from build123d import *

# Parameters (mm, degrees)
SKETCH1_R           = 8.75
BOSS_EXTRUDE1_DEPTH = 180
SKETCH2_R           = 8.75
SKETCH2_R_2         = 8
CUT_EXTRUDE1_DEPTH  = 40.95
CUT_EXTRUDE2_DEPTH  = 33.8
CUT_EXTRUDE3_DEPTH  = 33.8
CUT_EXTRUDE4_DEPTH  = 33.8
SKETCH7_R           = 8.75
BOSS_EXTRUDE2_DEPTH = 7.8
SKETCH9_R           = 8.75
BOSS_EXTRUDE3_DEPTH = 0.3
BOSS_EXTRUDE3_TAPER = 75


with BuildPart() as part:
    # Sketch1 → Boss-Extrude1 (new body)
    with BuildSketch(Plane.XY):
        Circle(SKETCH1_R)
    extrude(amount=BOSS_EXTRUDE1_DEPTH)

    # Sketch2 → Cut-Extrude1 (cut)
    with BuildSketch(Plane.XY.offset(180)):
        Circle(SKETCH2_R)
        Circle(SKETCH2_R_2, mode=Mode.SUBTRACT)
    cut_extrude1 = extrude(amount=-CUT_EXTRUDE1_DEPTH, mode=Mode.SUBTRACT)

    # Sketch3 → Cut-Extrude2 (cut)
    with BuildSketch(Plane.XY.offset(180)):
        with BuildLine():
            Line((-2.423043871, 5.999555366), (2.276956129, 5.999555366))
            Line((2.276956129, 5.999555366), (2.276956129, 7.669124513))
            ThreePointArc((2.276956129, 7.669124513), (-0.076415462, 7.999635034), (-2.423043871, 7.62422838))
            Line((-2.423043871, 7.62422838), (-2.423043871, 5.999555366))
        make_face()
    cut_extrude2 = extrude(amount=-CUT_EXTRUDE2_DEPTH, mode=Mode.SUBTRACT)

    # Sketch4 → Cut-Extrude3 (cut)
    with BuildSketch(Plane(origin=(0, 5.999555366, 0), x_dir=(1, 0, 0), z_dir=(0, 1, 0))):
        with BuildLine():
            Line((-2.423043871, -146.2), (2.276956129, -146.2))
            ThreePointArc((2.276956129, -146.2), (-0.073043871, -143.85), (-2.423043871, -146.2))
        make_face()
    cut_extrude3 = extrude(amount=CUT_EXTRUDE3_DEPTH, mode=Mode.SUBTRACT)

    # Mirror1: Cut-Extrude1, Cut-Extrude2, Cut-Extrude3 across plane
    add(cut_extrude1.mirror(Plane.XY.offset(90)), mode=Mode.SUBTRACT)
    add(cut_extrude2.mirror(Plane.XY.offset(90)), mode=Mode.SUBTRACT)
    add(cut_extrude3.mirror(Plane.XY.offset(90)), mode=Mode.SUBTRACT)

    # Sketch6 → Cut-Extrude4 (cut)
    with BuildSketch(Plane(origin=(0, 6.75, 0), x_dir=(1, 0, 0), z_dir=(0, 1, 0))):
        with BuildLine():
            Line((-2.35, -97), (-2.35, -83))
            ThreePointArc((-2.35, -83), (0, -80.65), (2.35, -83))
            Line((2.35, -83), (2.35, -97))
            ThreePointArc((2.35, -97), (0, -99.35), (-2.35, -97))
        make_face()
    extrude(amount=CUT_EXTRUDE4_DEPTH, mode=Mode.SUBTRACT)

    # Sketch7 → Boss-Extrude2 (add)
    with BuildSketch(Plane(origin=(0, 0, 40.95), x_dir=(-1, 0, 0), z_dir=(0, 0, -1))):
        Circle(SKETCH7_R)
    extrude(amount=-BOSS_EXTRUDE2_DEPTH)

    # Sketch9 → Boss-Extrude3 (add)
    with BuildSketch(Plane(origin=(0, 0, 40.95), x_dir=(-1, 0, 0), z_dir=(0, 0, -1))):
        Circle(SKETCH9_R)
    boss_extrude3 = extrude(amount=BOSS_EXTRUDE3_DEPTH, taper=BOSS_EXTRUDE3_TAPER)

    # Mirror4: Boss-Extrude3 across plane
    add(boss_extrude3.mirror(Plane.XY.offset(90)))


solid = part.part
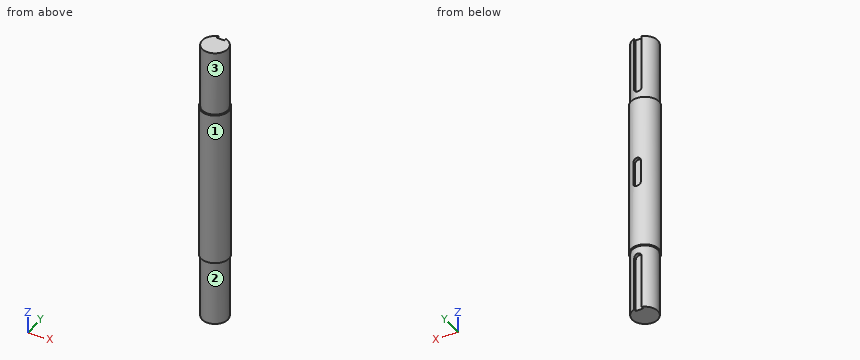
Part model, mm, in its own coordinate system. Face numbers are marked on the shaded views. A direction names the side the tool comes from. Give positions to 0.01 mm unless a question says otherwise; leave off trailing zeros. Order: outer loops, then holes, each group sorted by start corner. A loop starts at its lowest first (then second) coordinate and runs counter-clockwise, first axis right, second up. Notation, with made-up numbers: (33, -34.75) -> (46, -34.75) arc R22 cw to (46, 0.25) -> close; hole circle Ø7 at (35, 22). An arc over 180 degrees is marked (long way). Use one line per item in the form item = value.
(1) Saw through at C-C (z = 142). Write the cut outline in (x, y).
Solution:
outline = circle Ø16 at (0, 0)
(2) Drill centre lines: line 1 (Y direction, x = -0.5, z = 85); line 2 (Y direction, x = 0, z = 156); line 3 (X direction, y = 0.5, z = 154). Where is each one in solid material? Low to high. Write a range as from..to.
Solution:
line_1 = -8.74..6.75
line_2 = -8..6
line_3 = -7.98..7.98
(3) Saw through at B-B (z = 58). Write the cut outline in (x, y), then the cut area to 3 significant figures.
Solution:
outline = circle Ø17.5 at (0, 0)
area = 241 mm²
(4) Saw through at A-A (z = 87.5). Write the cut outline in (x, y).
Solution:
outline = (-2.35, 6.75) -> (-2.35, 8.43) arc R8.75 ccw (long way) to (2.35, 8.43) -> (2.35, 6.75) -> close
(5) Flat gauge pins, fed straight in: P1, Ø5, axis at x = 0, z = 90.5, coming from the +Y side; P2, Ø0.8, axis at y = 7, z = 21, coming from the +X side; P3, Ø1, axis at x = 3, z = 56.5, coming from the -Y side. Where does each tip first touch, or does it go through?
Solution:
P1 = 8.43
P2 = 4.52
P3 = -8.39
(6) Tool access for the marked faces 1, 2 and 3: list every direction of +Z, -Z, +X, -X, +Y, -Y with a clear straight run to the whole face (end or side of a thin tool).
Solution:
face_1 = +Z, -Z
face_2 = -Z
face_3 = +Z
